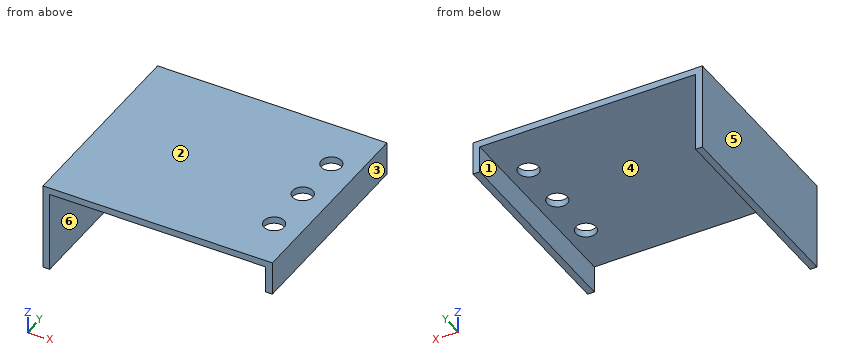
```python
from build123d import *

# Parameters (mm, degrees)
F0_W     = 215.9
F0_H     = 190.5
F1_DEPTH = 6.35
F2_R     = 9.525
F3_DEPTH = 25.4
F4_W     = 6.35
F4_H     = 190.5
F5_DEPTH = 76.2
F6_W     = 6.35
F6_H     = 190.5
F7_DEPTH = 25.4


with BuildPart() as f1:
    # F0 (on Top) → F1 (new body)
    with BuildSketch(Plane.XY):
        with Locations((41.449627, 35.641044)):
            Rectangle(F0_W, F0_H)
    extrude(amount=F1_DEPTH)

    # F2 (on face) → F3 (cut)
    with BuildSketch(Plane.XY.offset(6.35)):
        with Locations((123.999627, 83.266044)):
            Circle(F2_R)
        with Locations((123.999627, 35.641044)):
            Circle(F2_R)
        with Locations((123.999627, -11.983956)):
            Circle(F2_R)
    extrude(amount=-F3_DEPTH, mode=Mode.SUBTRACT)

    # F4 (on face) → F5 (join)
    with BuildSketch(Plane(origin=(0, 0, 0), x_dir=(1, 0, 0), z_dir=(0, 0, -1))):
        with Locations((-63.325373, -35.641044)):
            Rectangle(F4_W, F4_H)
    extrude(amount=F5_DEPTH)

    # F6 (on face) → F7 (join)
    with BuildSketch(Plane(origin=(0, 0, 0), x_dir=(1, 0, 0), z_dir=(0, 0, -1))):
        with Locations((146.224627, -35.641044)):
            Rectangle(F6_W, F6_H)
    extrude(amount=F7_DEPTH)


solid = f1.part
```
Source: CAD feature listing. Evaluate the final solid. Frame: model axes, mm. Face numbers are marked on the shaded views. A direction names the side the tool comes from. Give positions to 0.01 mm unless a question says otherwise; leave off trailing zeros. Write each loop counter-clockwise with the first axis right and the second up, starting at its lowest first coordinate (ties: lowest second). Pieces come first, ordered by that corner, then holes.
1. Section query C-C (y = 108.5). Return the cut outline in (x, z), then the cut area to 3 significant figures.
2. Section query D-D (x = -38.5). Return the cut outline in (y, z), then the cut area to 3 significant figures.
3. Material intervals for line 1 along X through (y, z) = (-17, -6); line 2 along X through (y, z) = (111, -64); line 3 along Z through (x, y) = (75.5, 12), sorted ascending.
4. Section query B-B (y = 41). Return the cut outline in (x, z).
5. Access query for the marked faces 5 and 6. Directions: +Z, -Z, +X, -X, +Y, -Y. A direction counts if a zero-diameter tool reaches every point of the face in a straight line with its end or side. Return the directions, or none.
6. Section query A-A (z = -16). Return the cut outline in (x, y).
7. First-contact query: pin 1 (12 mm diameter, centred on x = 115, y = 57, fed in from -Z); pin 2 (11.5 mm diameter, centred on x = 124, y = 35.64, fed in from +Z); pin 3 (1.9 mm diameter, centred on x = 147, y = 47, fed in from -Z); pin 4 (2 mm diameter, centred on y = 0.5, z = -34, fed in from +X). Flat tips, straight axial feed; report the tip coordinate or a pass-through.
8. Pull-direction query (X, two-part tool) for the marked faces 1, 2, 3 and 4; classes: +X half, -X half, draft (parallel to the pull), parting line (faces both ways), or undercut.
Output values:
1. outline: (-66.5, -76.2) - (-60.15, -76.2) - (-60.15, 0) - (143.05, 0) - (143.05, -25.4) - (149.4, -25.4) - (149.4, 6.35) - (-66.5, 6.35) - close
1. area: 2,020 mm2
2. outline: (-59.61, 0) - (130.89, 0) - (130.89, 6.35) - (-59.61, 6.35) - close
2. area: 1,210 mm2
3. line 1: x = -66.5 to -60.15, 143.05 to 149.4
3. line 2: x = -66.5 to -60.15
3. line 3: z = 0 to 6.35
4. outline: (-66.5, -76.2) - (-60.15, -76.2) - (-60.15, 0) - (116.13, 0) - (116.13, 6.35) - (-66.5, 6.35) - close; (131.87, 0) - (143.05, 0) - (143.05, -25.4) - (149.4, -25.4) - (149.4, 6.35) - (131.87, 6.35) - close
5. face 5: +Z, -Z, -X, +Y, -Y
5. face 6: -Z, +Y, -Y
6. outline: (-66.5, -59.61) - (-60.15, -59.61) - (-60.15, 130.89) - (-66.5, 130.89) - close; (143.05, -59.61) - (149.4, -59.61) - (149.4, 130.89) - (143.05, 130.89) - close
7. pin 1: stops at z = 0
7. pin 2: passes through
7. pin 3: stops at z = -25.4
7. pin 4: stops at x = -60.15
8. face 1: undercut
8. face 2: draft
8. face 3: +X half
8. face 4: undercut
